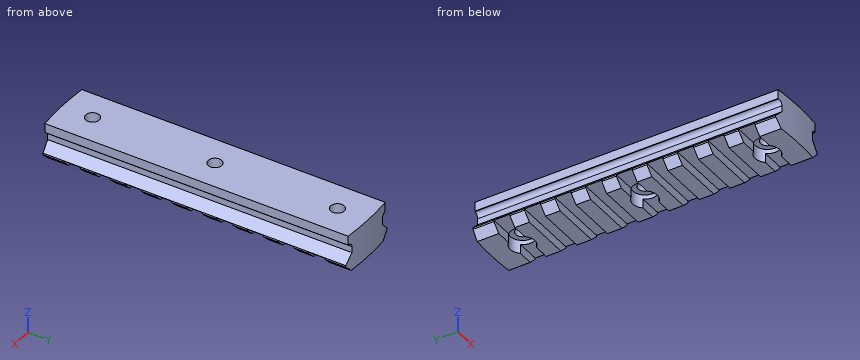
from build123d import *

# Parameters (mm, degrees)
BOSS_EXTRUDE1_DEPTH                                 = 50
SKETCH2_W                                           = 5
SKETCH2_H                                           = 5.25
CUT_EXTRUDE1_DEPTH                                  = 50
LPATTERN1_COUNT                                     = 5
LPATTERN1_PITCH                                     = 10
LPATTERN1_COL_COUNT                                 = 5
LPATTERN1_COL_PITCH                                 = 10
SKETCH3_OUTSIDE_W                                   = 43.794
SKETCH3_OUTSIDE_H                                   = 122.594
CUT_EXTRUDE2_DEPTH                                  = 50
CBORE_FOR_M4_HEX_SOCKET_HEAD_CAP_SCREW1_D           = 4.5
CBORE_FOR_M4_HEX_SOCKET_HEAD_CAP_SCREW1_CBORE_D     = 8
CBORE_FOR_M4_HEX_SOCKET_HEAD_CAP_SCREW1_CBORE_DEPTH = 4.4


with BuildPart() as part:
    # Sketch1 → Boss-Extrude1 (new, symmetric)
    with BuildSketch(Plane(origin=(0, 0, 0), x_dir=(1, 0, 0), z_dir=(0, 1, 0))):
        with BuildLine():
            Line((-8.07, 12.4), (8.07, 12.4))
            Line((8.07, 12.4), (10.6, 9.87))
            Line((10.6, 9.87), (10.6, 9.33))
            Line((10.6, 9.33), (7.8, 6.53))
            Line((7.8, 6.53), (7.8, 4.5))
            ThreePointArc((7.8, 4.5), (8.239339828, 3.439339828), (9.3, 3))
            Line((9.3, 3), (9.5, 3))
            Line((9.5, 3), (9.5, 0))
            Line((9.5, 0), (-9.5, 0))
            Line((-9.5, 0), (-9.5, 3))
            Line((-9.5, 3), (-9.3, 3))
            ThreePointArc((-9.3, 3), (-8.239339828, 3.439339828), (-7.8, 4.5))
            Line((-7.8, 4.5), (-7.8, 6.53))
            Line((-7.8, 6.53), (-10.6, 9.33))
            Line((-10.6, 9.33), (-10.6, 9.87))
            Line((-10.6, 9.87), (-8.07, 12.4))
        make_face()
    extrude(amount=BOSS_EXTRUDE1_DEPTH, both=True)

    # Sketch2 → Cut-Extrude1 (cut, symmetric)
    with BuildSketch(Plane(origin=(0, 0, 0), x_dir=(0, 0, -1), z_dir=(1, 0, 0))):
        with Locations((11.9, 0)):
            Rectangle(SKETCH2_W, SKETCH2_H)
    cut_extrude1 = extrude(amount=CUT_EXTRUDE1_DEPTH, both=True, mode=Mode.SUBTRACT)

    # LPattern1: Cut-Extrude1 ×5
    with Locations(*[(0, i * LPATTERN1_PITCH, 0) for i in range(1, LPATTERN1_COUNT)]):
        add(cut_extrude1, mode=Mode.SUBTRACT)

    # LPattern1 col: Cut-Extrude1 ×5
    with Locations(*[(0, -i * LPATTERN1_COL_PITCH, 0) for i in range(1, LPATTERN1_COL_COUNT)]):
        add(cut_extrude1, mode=Mode.SUBTRACT)

    # Sketch3 outside → Cut-Extrude2 (cut, symmetric)
    with BuildSketch(Plane.XY):
        Rectangle(SKETCH3_OUTSIDE_W, SKETCH3_OUTSIDE_H)
        with BuildLine():
            Line((-15, 48.868599666), (-15, -48.868599666))
            ThreePointArc((-15, -48.868599666), (0, -50), (15, -48.868599666))
            Line((15, -48.868599666), (15, 48.868599666))
            ThreePointArc((15, 48.868599666), (0, 50), (-15, 48.868599666))
        make_face(mode=Mode.SUBTRACT)
    extrude(amount=CUT_EXTRUDE2_DEPTH, both=True, mode=Mode.SUBTRACT)

    # CBORE for M4 Hex Socket Head Cap Screw1 (through all)
    with Locations(Plane(origin=(0, 0, -12.4), x_dir=(-1, 0, 0), z_dir=(0, 0, -1))):
        with Locations((0, 40), (0, -40), (0, 0)):
            CounterBoreHole(CBORE_FOR_M4_HEX_SOCKET_HEAD_CAP_SCREW1_D / 2, CBORE_FOR_M4_HEX_SOCKET_HEAD_CAP_SCREW1_CBORE_D / 2, CBORE_FOR_M4_HEX_SOCKET_HEAD_CAP_SCREW1_CBORE_DEPTH)


solid = part.part
Geometry check sheet. Reference: the model listing, model coordinates, mm. Round coordinates to 2 decimals unless told otherwise and drop trailing zeros. Write each loop counter-clockwise with the first axis right and the second up, starting at its lowest first coordinate (ties: lowest second). Pieces come first, ordered by that corner, then holes. Notation, with made-up numbers: (-10, 53) -> (36, 53) arc R25 cw to (36, 78) -> close; hole circle Ø11 at (12, 81.5). An arc over 180 degrees is marked (long way). One line per item, written item: value. Start each with the question number.
(1) Cross-section at A-A, the plane y = 0. Record the cut outline in (x, z).
(2) Scan lines: line 1 (Y direction, x = 0, z = -1.75); line 2 (Y direction, x = -7.75, z = -7.75); line 3 (Z direction, x = 2.5, y = 20). Record each from-to range of solid material in increasing order. Write a range as [from, to].
(3) Go/stop test with flat-tipped pins: pin 1 Ø3 at (y, z) = (29.5, -3) entering from -X; pin 2 Ø2.5 at (x, z) = (8, -10.5) entering from +Y; pin 3 Ø3.5 at (x, z) = (-4.5, -11) entering from +Y. Record where each tip stops, or that it passes through.
(4) Cross-section at C-C, the plane x = 0. Give the number of separate pieces and of enclosed holes in the cut face, and give its area (3 significant figures).
(5) Cross-section at B-B, the plane z = -1. Record the cut outline in (x, y).
(6) Cross-section at D-D, the plane y = 10.5. Record the cut outline in (x, z).
Answer:
1. outline: (-10.6, -9.4) -> (-4, -9.4) -> (-4, -8) -> (-2.25, -8) -> (-2.25, 0) -> (-9.5, 0) -> (-9.5, -3) -> (-9.3, -3) arc R1.5 cw to (-7.8, -4.5) -> (-7.8, -6.53) -> (-10.6, -9.33) -> close; (2.25, -8) -> (4, -8) -> (4, -9.4) -> (10.6, -9.4) -> (10.6, -9.33) -> (7.8, -6.53) -> (7.8, -4.5) arc R1.5 cw to (9.3, -3) -> (9.5, -3) -> (9.5, 0) -> (2.25, 0) -> close
2. line 1: [-50, -42.25], [-37.75, -2.25], [2.25, 37.75], [42.25, 50]
2. line 2: [-49.7, 49.7]
2. line 3: [-9.4, 0]
3. pin 1: x = -9.5
3. pin 2: y = 49.77
3. pin 3: y = 49.96
4. separate pieces: 4
4. enclosed holes: 0
4. area: 932 mm²
5. outline: (-9.5, -49.55) arc R100 ccw to (9.5, -49.55) -> (9.5, 49.55) arc R100 ccw to (-9.5, 49.55) -> close; hole circle Ø4.5 at (0, -40); hole circle Ø4.5 at (0, 0); hole circle Ø4.5 at (0, 40)
6. outline: (-10.6, -9.4) -> (10.6, -9.4) -> (10.6, -9.33) -> (7.8, -6.53) -> (7.8, -4.5) arc R1.5 cw to (9.3, -3) -> (9.5, -3) -> (9.5, 0) -> (-9.5, 0) -> (-9.5, -3) -> (-9.3, -3) arc R1.5 cw to (-7.8, -4.5) -> (-7.8, -6.53) -> (-10.6, -9.33) -> close
